```python
from build123d import *

# Parameters (mm, degrees)
CUT_EXTRUDE1_DEPTH = 12.506154875
CIRPATTERN1_COUNT  = 15


with BuildPart() as part:
    # Sketch1 → Revolve1 (revolve)
    with BuildSketch(Plane.XY, mode=Mode.PRIVATE) as revolve1_sk:
        Polygon((0, 0.5), (4.46, 0.5), (4.46, 7.5), (3.5, 7.5), (3.5, 1.75), (0, 1.75), align=None)
    revolve(revolve1_sk.sketch.rotate(Axis((-1851.483850706, 0, 0), (1, 0, 0)), 90), axis=Axis((-1851.483850706, 0, 0), (1, 0, 0)))

    # Sketch2 → Cut-Extrude1 (cut, through all)
    with BuildSketch(Plane(origin=(4.46, 0, 0), x_dir=(0, 0, -1), z_dir=(1, 0, 0))):
        with BuildLine():
            Line((-0.42512034, 6.486083001), (-0.179858605, 2.744112039))
            ThreePointArc((-0.179858605, 2.744112039), (0, 2.75), (0.179858605, 2.744112039))
            Line((0.179858605, 2.744112039), (0.42512034, 6.486083001))
            ThreePointArc((0.42512034, 6.486083001), (0, 6.5), (-0.42512034, 6.486083001))
        make_face()
    cut_extrude1 = extrude(amount=-CUT_EXTRUDE1_DEPTH, mode=Mode.SUBTRACT)

    # CirPattern1: Cut-Extrude1 ×15 about axis
    cirpattern1_axis = Axis((0, 0, 0), (1, 0, 0))
    for i in range(1, CIRPATTERN1_COUNT):
        add(cut_extrude1.rotate(cirpattern1_axis, i * 360 / CIRPATTERN1_COUNT), mode=Mode.SUBTRACT)


solid = part.part
```
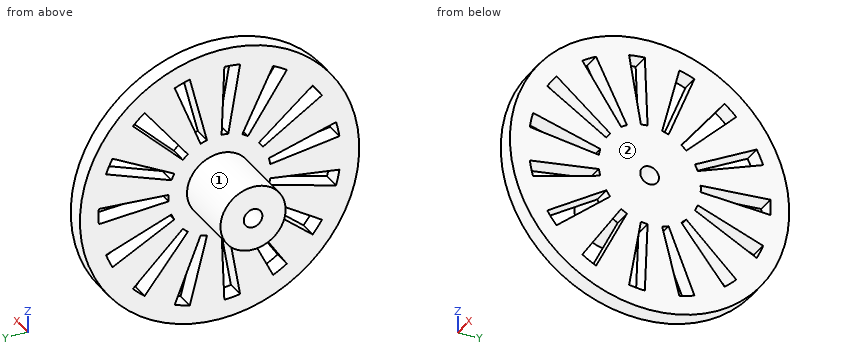
Could you check a few things on this model? Use its own coordinates, in mm. Face numbers are marked on the shaded views. Coordinates: 2 decimals unless noted, no trailing zeros. Write each loop counter-clockwise with the first axis right and the second up, starting at its lowest first coordinate (ties: lowest second). Pieces come first, ordered by that corner, then holes. Notation, with made-up numbers: M -18.75,52.5 L 38.25,52.5 A24 cw 38.25,65.5 Z; hole C 14,66.25 d1. An arc over 180 degrees is marked long. Answer as CSV lines item,"result". Start each with the question number.
1) For P1, Ø1, axis at x = 1, y = 1.5, coming from the -Z side; P2, Ø2, axis at x = 3, z = 4.5, coming from the -Y side; P3, Ø1.5, axis at x = 3, z = -3, coming from the +Y side, each with a flat end and sliding along its axis, tell me the tip position at first contact or that it passes through.
2) I want a section at D-D, the plane x = 4.05. Give the number of separate pieces and of enclosed holes in the cut face, and give its area (3 significant figures).
3) I want a section at B-B, the plane x = 2. Please give me the cut outline in (y, z), and give its area (3 significant figures).
4) I want a section at A-A, the plane z = 0. Please give me the cut outline in (x, y).
5) I want a section at C-C, the plane y = -4.5. Please give me the cut outline in (x, z).
6) We'd pull the mould along Y, two halves only. Please class the marked faces 1 and 2: +Y half, -Y half, draft (parallel to the pull), parting line (faces both ways), or undercut.
7) Please list where these lines run through material, in increasing order: line 1 (Y direction, x = 1.35, z = 0); line 2 (X direction, y = -5.5, z = -1.75); line 3 (Z direction, x = 3.7, y = 5). Write a range as from..to.
Data:
1,P1,"stops at z = -1.44"
1,P2,"stops at y = -6.56"
1,P3,"stops at y = 7.09"
2,separate pieces,"1"
2,enclosed holes,"16"
2,area,"142 mm^2"
3,outline,"C 0,0 d3.5; hole C 0,0 d1"
3,area,"8.84 mm^2"
4,outline,"M 0,-1.75 L 3.5,-1.75 L 3.5,-7.5 L 4.46,-7.5 L 4.46,-0.5 L 0,-0.5 Z; M 0,0.5 L 4.46,0.5 L 4.46,2.75 L 3.5,2.75 L 3.5,1.75 L 0,1.75 Z; M 3.5,6.5 L 4.46,6.5 L 4.46,7.5 L 3.5,7.5 Z"
5,outline,"M 3.5,-6 L 4.46,-6 L 4.46,-3.74 L 3.5,-3.74 Z; M 3.5,-2.84 L 4.46,-2.84 L 4.46,-1.27 L 3.5,-1.27 Z; M 3.5,-0.65 L 4.46,-0.65 L 4.46,0.65 L 3.5,0.65 Z; M 3.5,1.27 L 4.46,1.27 L 4.46,2.84 L 3.5,2.84 Z; M 3.5,3.74 L 4.46,3.74 L 4.46,6 L 3.5,6 Z"
6,face 1,"parting line"
6,face 2,"draft"
7,line 1,"y = -1.75..-0.5, 0.5..1.75"
7,line 2,"x = 3.5..4.46"
7,line 3,"z = -5.59..-2.63, -1.84..-0.33, 0.33..1.84, 2.63..5.59"
